Input: part model. Units: mm. Frame: model coordinates. Face numbers are marked on the shaded views. A direction names the side the tool comes from. Coordinates: 2 decimals unless noted, no trailing zeros. Write each loop counter-clockwise with the first axis right and the second up, starting at its lowest first coordinate (ties: lowest second). Pieces come first, ordered by that corner, then holes.
1) Section query A-A (y = 0). Output: boundary loops of the cut face in (x, z).
2) Section query B-B (x = 0). Output: boundary loops of the cut face in (y, z).
3) Draft query along Y for the marked faces 5, 6 and 7. Return one class per face: pulls with the +Y half, pulls with the -Y half, needs draft (parallel to the pull), parting line crosses it, or undercut.
4) Line query: L1, parallel to X at y = -1.75, z = -2.7; L2, parallel to Y at x = 0.5, z = -2.9; L3, parallel to Z at x = 2.5, y = -1.75. Output: solid intervals per line, ascending.
5) Set-up query: the marked faces 1, 2, 3 and 4. Return all of +Z, -Z, +X, -X, +Y, -Y with unobstructed straight access to the full face (end or side cutting, diameter ignored); none if empty.
6) Pin query (flat end, axial travel): pin 1 Ø1.1 at (y, z) = (3.5, -2.5) entering from -X; pin 2 Ø0.7 at (y, z) = (-3, -2.5) entering from +X; pin 3 Ø0.5 at (x, z) = (-4, -2.5) entering from +Y; pin 4 Ø0.8 at (x, z) = (-4.5, -2.5) entering from -Y. Return the tip coordinate at first contact, or that it passes through.
7) Section query C-C (z = -3.25). Output: boundary loops of the cut face in (x, y).
8) Section query D-D (y = -1.75). Output: boundary loops of the cut face in (x, z), then the cut area to 3 significant figures.
from build123d import *

# Parameters (mm, degrees)
F1_DEPTH = 2.6
F3_DEPTH = 3.5
F5_D     = 2.4


with BuildPart() as f1:
    # F0 (on Front) → F1 (new body, symmetric)
    with BuildSketch(Plane.XZ):
        with BuildLine():
            Line((-3.6, -0.35), (3.6, -0.35))
            ThreePointArc((3.6, -0.35), (4.0949747468, -0.5550252532), (4.3, -1.05))
            Line((4.3, -1.05), (4.3, -3.65))
            Line((4.3, -3.65), (5, -3.65))
            Line((5, -3.65), (5, -1.05))
            ThreePointArc((5, -1.05), (4.5899494937, -0.0600505063), (3.6, 0.35))
            Line((3.6, 0.35), (-3.6, 0.35))
            ThreePointArc((-3.6, 0.35), (-4.5899494937, -0.0600505063), (-5, -1.05))
            Line((-5, -1.05), (-5, -3.65))
            Line((-5, -3.65), (-4.3, -3.65))
            Line((-4.3, -3.65), (-4.3, -1.05))
            ThreePointArc((-4.3, -1.05), (-4.0949747468, -0.5550252532), (-3.6, -0.35))
        make_face()
    extrude(amount=F1_DEPTH, both=True)

    # F2 (on Right) → F3 (join, symmetric)
    with BuildSketch(Plane.YZ):
        with BuildLine():
            Line((-4, -3.65), (-3.3, -3.65))
            Line((-3.3, -3.65), (-3.3, -1.05))
            ThreePointArc((-3.3, -1.05), (-3.0949747468, -0.5550252532), (-2.6, -0.35))
            Line((-2.6, -0.35), (-2.6, 0.35))
            ThreePointArc((-2.6, 0.35), (-3.5899494937, -0.0600505063), (-4, -1.05))
            Line((-4, -1.05), (-4, -3.65))
        make_face()
        with BuildLine():
            ThreePointArc((4, -1.05), (3.5899494937, -0.0600505063), (2.6, 0.35))
            Line((2.6, 0.35), (2.6, -0.35))
            ThreePointArc((2.6, -0.35), (3.0949747468, -0.5550252532), (3.3, -1.05))
            Line((3.3, -1.05), (3.3, -3.65))
            Line((3.3, -3.65), (4, -3.65))
            Line((4, -3.65), (4, -1.05))
        make_face()
    extrude(amount=F3_DEPTH, both=True)

    # F5 (through all)
    with Locations(Plane.XY.offset(0.35)):
        with Locations((0, 0)):
            Hole(F5_D / 2)


solid = f1.part
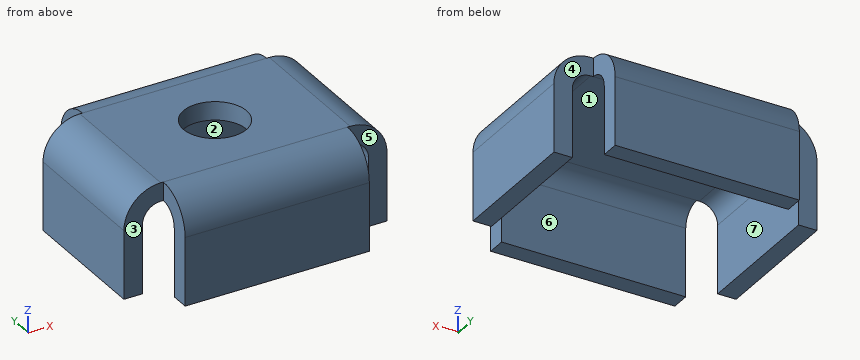
Answer:
1. outline: (-5, -3.65) - (-4.3, -3.65) - (-4.3, -1.05) arc R0.7 cw to (-3.6, -0.35) - (-1.2, -0.35) - (-1.2, 0.35) - (-3.6, 0.35) arc R1.4 ccw to (-5, -1.05) - close; (1.2, -0.35) - (3.6, -0.35) arc R0.7 cw to (4.3, -1.05) - (4.3, -3.65) - (5, -3.65) - (5, -1.05) arc R1.4 ccw to (3.6, 0.35) - (1.2, 0.35) - close
2. outline: (-4, -3.65) - (-3.3, -3.65) - (-3.3, -1.05) arc R0.7 cw to (-2.6, -0.35) - (-1.2, -0.35) - (-1.2, 0.35) - (-2.6, 0.35) arc R1.4 ccw to (-4, -1.05) - close; (1.2, -0.35) - (2.6, -0.35) arc R0.7 cw to (3.3, -1.05) - (3.3, -3.65) - (4, -3.65) - (4, -1.05) arc R1.4 ccw to (2.6, 0.35) - (1.2, 0.35) - close
3. face 5: pulls with the -Y half
3. face 6: undercut
3. face 7: needs draft
4. L1: x = -5 to -4.3, 4.3 to 5
4. L2: y = -4 to -3.3, 3.3 to 4
4. L3: z = -0.35 to 0.35
5. face 1: -Z
5. face 2: -Z, +X, -X
5. face 3: +Z, -Z, -X, -Y
5. face 4: +Z, -Z, +X, +Y
6. pin 1: stops at x = -3.5
6. pin 2: stops at x = 3.5
6. pin 3: passes through
6. pin 4: stops at y = -2.6
7. outline: (-5, -2.6) - (-4.3, -2.6) - (-4.3, 2.6) - (-5, 2.6) - close; (-3.5, -4) - (3.5, -4) - (3.5, -3.3) - (-3.5, -3.3) - close; (-3.5, 3.3) - (3.5, 3.3) - (3.5, 4) - (-3.5, 4) - close; (4.3, -2.6) - (5, -2.6) - (5, 2.6) - (4.3, 2.6) - close
8. outline: (-5, -3.65) - (-4.3, -3.65) - (-4.3, -1.05) arc R0.7 cw to (-3.6, -0.35) - (3.6, -0.35) arc R0.7 cw to (4.3, -1.05) - (4.3, -3.65) - (5, -3.65) - (5, -1.05) arc R1.4 ccw to (3.6, 0.35) - (-3.6, 0.35) arc R1.4 ccw to (-5, -1.05) - close
8. area: 11.0 mm2
